Design review of the part shown in the three views and the two pictorial views. Dimensions are in mm from the part's minimum x, y and z. A direction names the side the tool comes from. Coordinates: 2 decimals unless noted, no trailing zeros. Order: outer loops, then holes, each group sorted by start corner. A loop starts at its lowest first (then second) coordinate and runs counter-clockwise, first axis right, second up. Notation, with made-up numbers: (64.5, 33.5) -> (99.5, 33.5) arc R17 cw to (99.5, 45.5) -> close; hole circle Ø5 at (70.5, -7). An arc over 180 degrees is marked (long way). Answer as a JSON object with one key per item and string values. Group by question number.
1) Machinability: for the marked faces 1 and 2, which of the approach directions +Z, -Z, +X, -X, +Y, -Y give a long, thin tool a straight path to every point of the face, cutting with its end or side? Answer none if there is none.
2) Add section C-C, the plane y = 2. Write out the cut boundary in (x, z).
3) Add section A-A, the plane z = 23. Write out the cut boundary in (x, y), then the cut area to 3 significant figures.
4) Add section B-B, the plane x = 23. Write out the cut boundary in (y, z).
5) Add section D-D, the plane z = 14.5. Write out the cut boundary in (x, y), then the cut area to 3 significant figures.
6) For pin 1 (2 mm diameter, centred on x = 21, y = 3.5, fed in from +Z) (3 decimals); pin 2 (1 mm diameter, centred on x = 25, y = 6, fed in from -Z); pin 3 (3 mm diameter, centred on x = 37, y = 1, fed in from -Z), all flat-tipped, find the tip position at first contact; note any pin that passes through.
7) Draft analysis for pull direction Z (two halves, no side actions). For the marked faces 3 and 4, state which applies: +Z half, -Z half, draft (parallel to the pull), parting line (faces both ways), or undercut.
8) Wall thickness on L1, parallel to X at y = 4.75, z = 23; L2, parallel to Y at x = 10, z = 40; L3, parallel to X at y = 3, z = 21: over which ranges is each line inside the solid? List them lowest first.
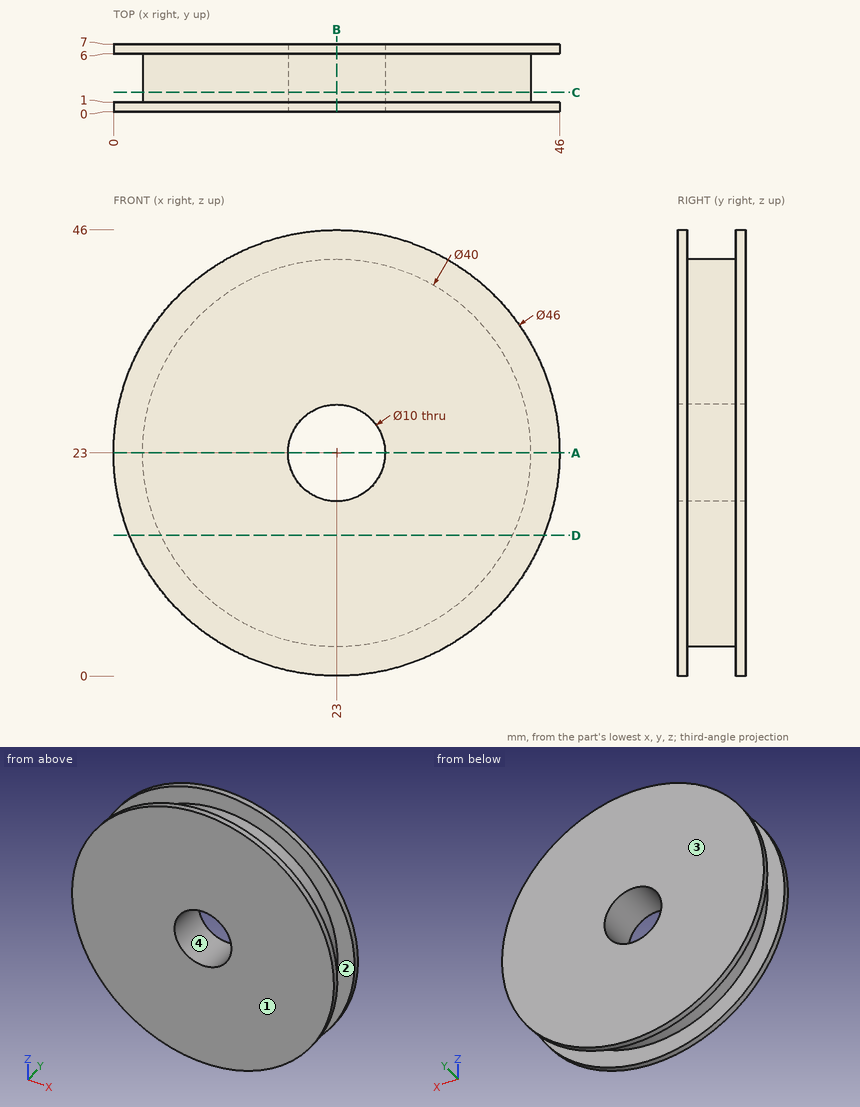
Output values:
{
 "1": {"face 1": "+Z, -Z, +X, -X, -Y", "face 2": "none"},
 "2": {"outline": "circle Ø40 at (23, 23); hole circle Ø10 at (23, 23)"},
 "3": {"outline": "(0, 0) -> (18, 0) -> (18, 7) -> (0, 7) -> (0, 6) -> (3, 6) -> (3, 1) -> (0, 1) -> close; (28, 0) -> (46, 0) -> (46, 1) -> (43, 1) -> (43, 6) -> (46, 6) -> (46, 7) -> (28, 7) -> close", "area": "222 mm²"},
 "4": {"outline": "(0, 0) -> (1, 0) -> (1, 3) -> (6, 3) -> (6, 0) -> (7, 0) -> (7, 18) -> (0, 18) -> close; (0, 28) -> (7, 28) -> (7, 46) -> (6, 46) -> (6, 43) -> (1, 43) -> (1, 46) -> (0, 46) -> close"},
 "5": {"outline": "(1.63, 0) -> (44.37, 0) -> (44.37, 1) -> (41.1, 1) -> (41.1, 6) -> (44.37, 6) -> (44.37, 7) -> (1.63, 7) -> (1.63, 6) -> (4.9, 6) -> (4.9, 1) -> (1.63, 1) -> close", "area": "267 mm²"},
 "6": {"pin 1": "stops at z = 42.975", "pin 2": "stops at z = 0.05", "pin 3": "stops at z = 3.69"},
 "7": {"face 3": "draft", "face 4": "undercut"},
 "8": {"L1": "x = 3 to 18, 28 to 43", "L2": "y = 0 to 1, 6 to 7", "L3": "x = 3.1 to 18.42, 27.58 to 42.9"}
}
